Part print with two shaded views. Sizes in mm from the minimum x, y, z corner. A direction names the side the tool comes from. Round coordinates to 2 decimals unless told otherwise and drop trailing zeros. Order: outer loops, then holes, each group sorted by start corner. A loop starts at its lowest first (then second) coordinate and runs counter-clockwise, first axis right, second up. Notation, with made-up numbers: (52.25, -11) -> (66.25, -11) arc R13 ccw to (66.25, -4) -> close; hole circle Ø7 at (-17, 9). An arc over 180 degrees is marked (long way). Put each result on its own line as item: value. Start each with the question number.
Q1. 3-axis set-ups, long thin cutter, end or side, ignore diameter. For the marked faces 1, 2, 3 and 4: which of +Z, -Z, +X, -X, +Y, -Y reach the whole face in a straight line?
Q2. Pull direction Y, two halves, no side cores. Call the marked faces 5, 6 and 7: released by +Y, released by -Y, zero draft, split by the parting line, or undercut.
Q3. Cut at D-D, the plane y = 30. List the corners of the cut face in (x, z), and give its area (3 significant figures).
Q4. Probe L1, parallel to X at y = 24, z = 1.5; L2, parallel to Y at x = 16.5, z = 15.75. List the from-to ranges inside material, lowest first.
Q5. Cut at B-B, the plane y = 25. List the corners of the cut face in (x, z).
Q6. Cut at C-C, the plane z = 15.75. List the corners of the cut face in (x, y), and give its area (4 significant figures).
Q7. Cut at A-A, the plane x = 16.5. List the corners of the cut face in (y, z), and give its area (3 significant figures).
Q8. Flat gauge pins, fed straight in: P1, Ø2, axis at x = 26, y = 19, coming from the -Z side; P2, Ø4, axis at x = 14, y = 31, coming from the -Z side; P3, Ø2, axis at x = 16, y = 6.5, coming from the +Z side. Where does each tip first touch, or does it go through?
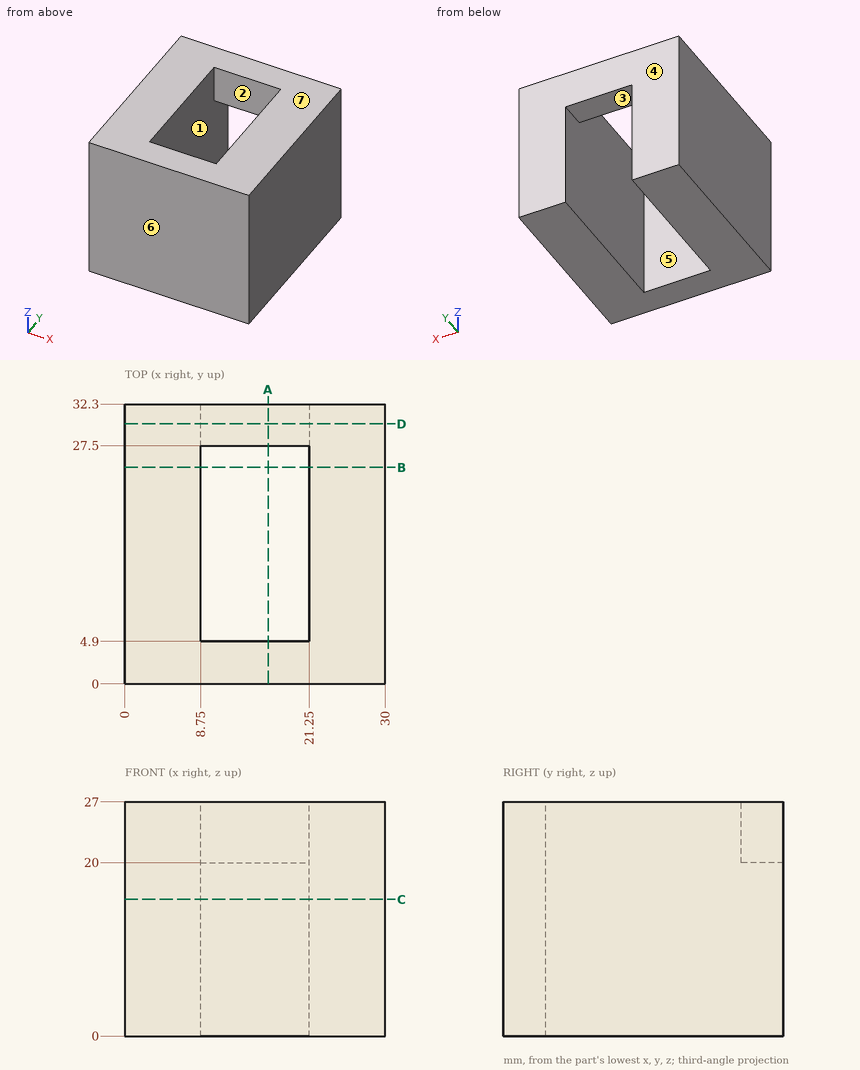
Ans:
1. face 1: -Z
1. face 2: +Z, -Z
1. face 3: -Z, +Y
1. face 4: +Z, -Z, +X, -X, +Y
2. face 5: undercut
2. face 6: released by -Y
2. face 7: zero draft
3. outline: (0, 0) -> (8.75, 0) -> (8.75, 20) -> (21.25, 20) -> (21.25, 0) -> (30, 0) -> (30, 27) -> (0, 27) -> close
3. area: 560 mm^2
4. L1: x = 0 to 8.75, 21.25 to 30
4. L2: y = 0 to 4.9
5. outline: (0, 0) -> (8.75, 0) -> (8.75, 27) -> (0, 27) -> close; (21.25, 0) -> (30, 0) -> (30, 27) -> (21.25, 27) -> close
6. outline: (0, 0) -> (30, 0) -> (30, 32.3) -> (21.25, 32.3) -> (21.25, 4.9) -> (8.75, 4.9) -> (8.75, 32.3) -> (0, 32.3) -> close
6. area: 626.5 mm^2
7. outline: (0, 0) -> (4.9, 0) -> (4.9, 27) -> (0, 27) -> close; (27.5, 20) -> (32.3, 20) -> (32.3, 27) -> (27.5, 27) -> close
7. area: 166 mm^2
8. P1: stops at z = 0
8. P2: stops at z = 20
8. P3: passes through
